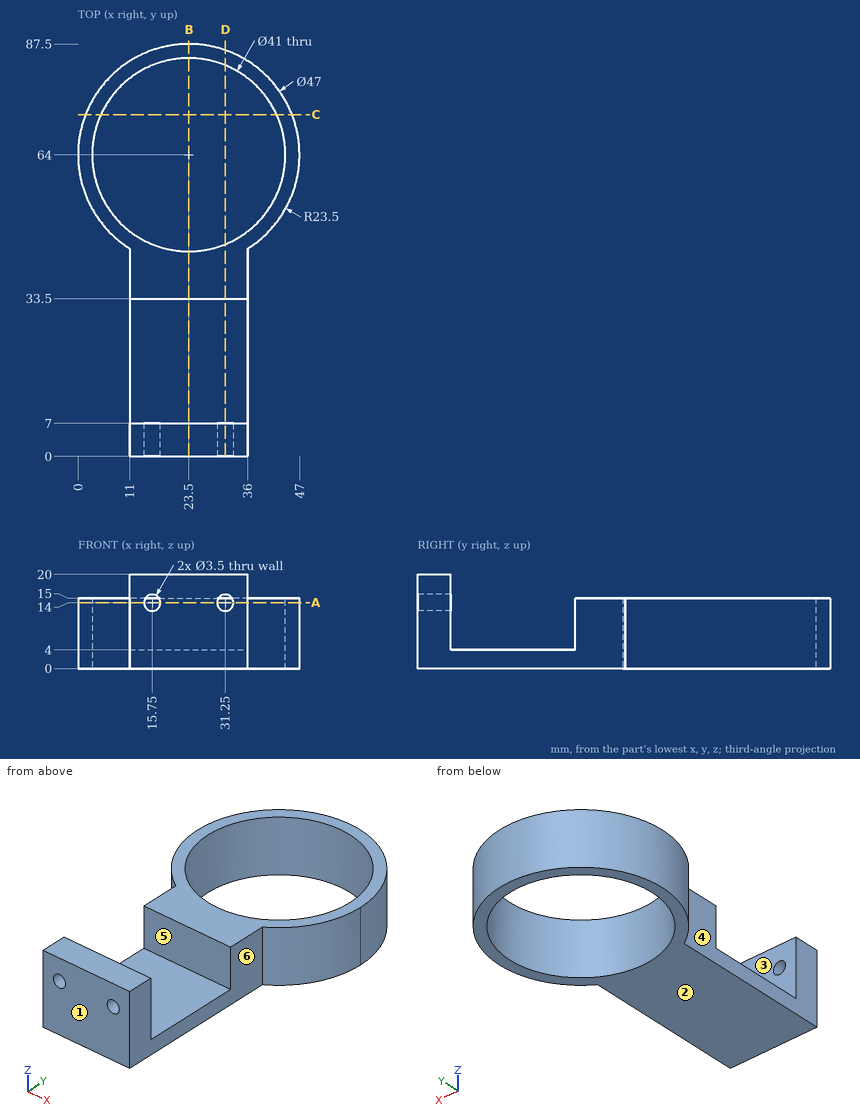
Can you work these out from the drawing? Everything is in mm from the part's minimum corner. A direction names the side the tool comes from. Round coordinates to 2 decimals unless told otherwise and drop trailing zeros. Loops run counter-clockwise (first coordinate to the right, second up) from the corner with the lowest first, then second, coordinate; pieces in that order, holes last. Notation, with made-up numbers: (52, -13.5) - (96, -13.5) arc R29 ccw to (96, 21.5) - close; hole circle Ø5 at (86.25, -11.5). An arc over 180 degrees is marked (long way). One line per question, with ' | ' between items. Start each with the question number.
Q1. I want a section at C-C (y = 72.5). Write out the boundary of the cut face in (x, z), then the cut area to 3 significant figures.
Q2. Will these pins go through, and if not, where does the flat tip stop? pin 1 (6 mm diameter, centred on y = 14.5, z = 8, fed in from +X); pin 2 (6 mm diameter, centred on x = 36, y = 13, fed in from +Z); pin 3 (3 mm diameter, centred on x = 31.25, z = 14, fed in from -Y); pin 4 (1.5 mm diameter, centred on x = 12.5, z = 2.5, fed in from +Y).
Q3. We'd pull the mould along Y, two halves only. Please class the marked faces 1, 2 and 3: +Y half, -Y half, draft (parallel to the pull), parting line (faces both ways), or undercut.
Q4. I want a section at D-D (x = 31.25). Write out the boundary of the cut face in (y, z), then the cut area to 3 significant figures.
Q5. I want a section at A-A (z = 14). Write out the boundary of the cut face in (x, y), then the cut area to 3 significant figures.
Q6. I want a section at B-B (x = 23.5). Write out the boundary of the cut face in (y, z), then the cut area to 3 significant figures.
Q7. Please list where these lines run through material, in increasing order: line 1 (Y direction, x = 23.5, z = 10); line 2 (Z direction, x = 15.75, y = 2.25); line 3 (Y direction, x = 16.5, z = 5). Write a range as [from, to].
Q8. For the marked faces 4, 5 and 6, which set-ups out of +Z, -Z, +X, -X, +Y, -Y let a thin tool reach every point of the face, with its end or its side?
Response values:
1) outline: (1.59, 0) - (4.85, 0) - (4.85, 15) - (1.59, 15) - close; (42.15, 0) - (45.41, 0) - (45.41, 15) - (42.15, 15) - close | area: 97.6 mm²
2) pin 1: passes through | pin 2: stops at z = 4 | pin 3: stops at y = 33.5 | pin 4: stops at y = 85.15
3) face 1: -Y half | face 2: draft | face 3: undercut
4) outline: (0, 0) - (45.02, 0) - (45.02, 15) - (33.5, 15) - (33.5, 4) - (7, 4) - (7, 12.25) - (0, 12.25) - close; (0, 15.75) - (7, 15.75) - (7, 20) - (0, 20) - close; (82.98, 0) - (86.19, 0) - (86.19, 15) - (82.98, 15) - close | area: 442 mm²
5) outline: (11, 0) - (14, 0) - (14, 7) - (11, 7) - close; (11, 33.5) - (36, 33.5) - (36, 44.1) arc R23.5 ccw (long way) to (11, 44.1) - close; (17.5, 0) - (29.5, 0) - (29.5, 7) - (17.5, 7) - close; (33, 0) - (36, 0) - (36, 7) - (33, 7) - close; hole circle Ø41 at (23.5, 64) | area: 745 mm²
6) outline: (0, 0) - (43.5, 0) - (43.5, 15) - (33.5, 15) - (33.5, 4) - (7, 4) - (7, 20) - (0, 20) - close; (84.5, 0) - (87.5, 0) - (87.5, 15) - (84.5, 15) - close | area: 441 mm²
7) line 1: y = [0, 7], [33.5, 43.5], [84.5, 87.5] | line 2: z = [0, 12.25], [15.75, 20] | line 3: y = [0, 7], [33.5, 44.73], [83.27, 86.43]
8) face 4: +Z, -Z, -X, -Y | face 5: +Z, +X, -X | face 6: +Z, -Z, +X, -Y
